The listing builds one solid part. Answer for the finished solid, in the listing's coordinates (mm). Face numbers are marked on the shaded views. A direction names the side the tool comes from. Round coordinates to 2 decimals unless told otherwise and drop trailing zeros. Loops run counter-clockwise (first coordinate to the right, second up) from the corner with the lowest first, then second, coordinate; pieces in that order, holes last. Notation, with made-up numbers: (72.25, 54) -> (93.25, 54) arc R16 ccw to (93.25, 85) -> close; hole circle Ø2 at (-37.5, 41). An arc over 180 degrees is marked (long way). One line per question, with ' | ' between items.
from build123d import *
from build123d.topology import SkipClean

# Parameters (mm, degrees)
SKETCH2_W                      = 63.5
SKETCH2_H                      = 63.5
BOSS_EXTRUDE1_DEPTH            = 80
CUT_EXTRUDE1_REACH             = 93.739
SKETCH4_R                      = 14.2875
CUT_EXTRUDE2_DEPTH             = 3.81
CUT_EXTRUDE3_DEPTH             = 62.22
CUT_EXTRUDE4_REACH             = 93.739
CUT_EXTRUDE4_DIRECTION_2_REACH = 93.739
FILLET2_R                      = 2.54
SKETCH9_W                      = 5
SKETCH9_H                      = 80
BOSS_EXTRUDE2_DEPTH            = 35
SKETCH10_R                     = 2.75
CUT_EXTRUDE6_DEPTH             = 119.642846392
CUT_EXTRUDE7_REACH             = 110.92
SKETCH11_R                     = 3
SKETCH12_W                     = 40
SKETCH12_H                     = 80
BOSS_EXTRUDE3_DEPTH            = 15
SKETCH13_R                     = 3
CUT_EXTRUDE8_DEPTH             = 10
FILLET3_R                      = 3.175
FILLET4_DEPTH                  = 80


with BuildPart() as part:
    # Sketch2 → Boss-Extrude1 (new body)
    with BuildSketch(Plane(origin=(0, 0, 0), x_dir=(1, 0, 0), z_dir=(0, 1, 0))):
        Rectangle(SKETCH2_W, SKETCH2_H)
    extrude(amount=BOSS_EXTRUDE1_DEPTH)

    # Sketch3 → Cut-Extrude1 (cut, up to next)
    with BuildSketch(Plane(origin=(0, 80, 0), x_dir=(1, 0, 0), z_dir=(0, 1, 0)), mode=Mode.PRIVATE) as cut_extrude1_sk1:
        with BuildLine():
            Line((9.525, 0), (14.2875, 0))
            ThreePointArc((14.2875, 0), (0, -14.2875), (-14.2875, 0))
            Line((-14.2875, 0), (-9.525, 0))
            ThreePointArc((-9.525, 0), (0, 9.525), (9.525, 0))
        make_face()
    cut_extrude1_tool1 = extrude(cut_extrude1_sk1.sketch, amount=-CUT_EXTRUDE1_REACH, mode=Mode.PRIVATE) & part.part
    add(cut_extrude1_tool1.solids().sort_by_distance((0, 80, 2.954161))[0], mode=Mode.SUBTRACT)

    # Sketch4 → Cut-Extrude2 (cut)
    with BuildSketch(Plane(origin=(0, 80, 0), x_dir=(1, 0, 0), z_dir=(0, 1, 0))):
        with Locations(Location((0, 0, 0), (0, 0, 270))):
            Circle(SKETCH4_R)
    extrude(amount=-CUT_EXTRUDE2_DEPTH, mode=Mode.SUBTRACT)

    # Sketch6 → Cut-Extrude3 (cut)
    with BuildSketch(Plane(origin=(0, 71.11, 0), x_dir=(1, 0, 0), z_dir=(0, 1, 0))):
        with BuildLine():
            Line((9.525, 0), (19.05, 31.75))
            Line((19.05, 31.75), (-19.05, 31.75))
            Line((-19.05, 31.75), (-9.525, 0))
            ThreePointArc((-9.525, 0), (0, 9.525), (9.525, 0))
        make_face()
    extrude(amount=-CUT_EXTRUDE3_DEPTH, mode=Mode.SUBTRACT)

    # Cut-Extrude4: up to this plane
    with SkipClean():  # the faces are left unmerged after this step: merging them gives an invalid solid
        cut_extrude4_end = Plane(origin=(-9.525, -49.595085442, 0), z_dir=(-0.9578262852211514, 0, 0.2873478855663456))
        # Sketch7 → Cut-Extrude4 (cut, up to the surface)
        with BuildSketch(Plane(origin=(0, 0, 0), x_dir=(0, 0, -1), z_dir=(1, 0, 0)), mode=Mode.PRIVATE) as cut_extrude4_sk1:
            Polygon((0, 8.89), (31.75, 8.89), (0, 0), align=None)
        cut_extrude4_tool1 = split(extrude(cut_extrude4_sk1.sketch, amount=-CUT_EXTRUDE4_REACH, mode=Mode.PRIVATE), bisect_by=cut_extrude4_end, keep=Keep.BOTH, mode=Mode.PRIVATE)
        add(cut_extrude4_tool1.solids().sort_by_distance((0, 5.926667, -10.583333))[0], mode=Mode.SUBTRACT)

    # Cut-Extrude4 direction 2: up to this plane
    cut_extrude4_direction_2_end = Plane(origin=(9.525, -49.595085442, 0), z_dir=(0.9578262852211514, 0, 0.2873478855663456))
    # Sketch7 → Cut-Extrude4 direction 2 (cut, up to the surface)
    with BuildSketch(Plane(origin=(0, 0, 0), x_dir=(0, 0, -1), z_dir=(1, 0, 0)), mode=Mode.PRIVATE) as cut_extrude4_direction_2_sk1:
        Polygon((0, 8.89), (31.75, 8.89), (0, 0), align=None)
    cut_extrude4_direction_2_tool1 = split(extrude(cut_extrude4_direction_2_sk1.sketch, amount=CUT_EXTRUDE4_DIRECTION_2_REACH, mode=Mode.PRIVATE), bisect_by=cut_extrude4_direction_2_end, keep=Keep.BOTH, mode=Mode.PRIVATE)
    add(cut_extrude4_direction_2_tool1.solids().sort_by_distance((0, 5.926667, -10.583333))[0], mode=Mode.SUBTRACT)

    # Fillet2
    # the kernel refuses this fillet: 2.54 mm, written as the material it adds along each edge
    with BuildSketch(Plane(origin=(7.700340927, 71.11, 6.082196911), x_dir=(-0.9578262852211513, 0, -0.2873478855663455), z_dir=(0.28734788556634555, 0, -0.9578262852211513))) as fillet2_piece_1_section:
        with BuildLine():
            CenterArc((FILLET2_R, -FILLET2_R), FILLET2_R, 90, 90)
            Line((0, -FILLET2_R), (0, 0))
            Line((0, 0), (FILLET2_R, 0))
        make_face()
    fillet2_piece_1 = extrude(amount=45.847973166, mode=Mode.PRIVATE)
    fillet2_piece_1 = split(fillet2_piece_1, bisect_by=Plane(origin=(7.700340927, 71.11, -31.75), z_dir=(0, 0, 1)), keep=Keep.TOP, mode=Mode.PRIVATE)
    fillet2_piece_1 = fillet2_piece_1 - Plane(origin=(0, 71.11, 0), x_dir=(-1, 0, 0), z_dir=(0, 1, 0)) * Cylinder(9.525, 102, mode=Mode.PRIVATE)
    fillet2_piece_1 = split(fillet2_piece_1, bisect_by=Plane(origin=(7.700340927, 71.11, 0), z_dir=(0, 0, -1)), keep=Keep.TOP, mode=Mode.PRIVATE)
    add(fillet2_piece_1)
    with BuildSketch(Plane(origin=(-20.874659073, 71.11, -37.832196911), x_dir=(0, -1, 0), z_dir=(0.28734788556634555, 0, 0.9578262852211513))) as fillet2_piece_2_section:
        with BuildLine():
            CenterArc((FILLET2_R, FILLET2_R), FILLET2_R, 180, 90)
            Line((0, FILLET2_R), (0, 0))
            Line((0, 0), (FILLET2_R, 0))
        make_face()
    fillet2_piece_2 = extrude(amount=45.847973166, mode=Mode.PRIVATE)
    fillet2_piece_2 = split(fillet2_piece_2, bisect_by=Plane(origin=(-20.874659073, 71.11, -31.75), z_dir=(0, 0, 1)), keep=Keep.TOP, mode=Mode.PRIVATE)
    fillet2_piece_2 = split(fillet2_piece_2, bisect_by=Plane(origin=(-20.874659073, 71.11, 0), z_dir=(0, 0, -1)), keep=Keep.TOP, mode=Mode.PRIVATE)
    fillet2_piece_2 = fillet2_piece_2 - Plane(origin=(0, 71.11, 0), x_dir=(-1, 0, 0), z_dir=(0, 1, 0)) * Cylinder(9.525, 102, mode=Mode.PRIVATE)
    add(fillet2_piece_2)
    with BuildSketch(Plane(origin=(-20.954648619, 10.667672044, -38.098828729), x_dir=(0.9607141016314922, 0.07483307171461691, -0.2672609704093551), z_dir=(0.2775399339309484, -0.2590372716688848, 0.9251331131031606))) as fillet2_piece_3_section:
        with BuildLine():
            CenterArc((FILLET2_R * 1.08072615035, FILLET2_R), FILLET2_R, 175.556407911, 94.443592089)
            Line((FILLET2_R * 0.0837320564804, FILLET2_R * 1.07747758898), (0, 0))
            Line((0, 0), (FILLET2_R * 1.08072615035, 0))
        make_face()
    fillet2_piece_3 = extrude(amount=52.848435405, mode=Mode.PRIVATE)
    fillet2_piece_3 = split(fillet2_piece_3, bisect_by=Plane(origin=(-20.954648619, 10.667672044, -31.75), z_dir=(0, 0, 1)), keep=Keep.TOP, mode=Mode.PRIVATE)
    fillet2_piece_3 = fillet2_piece_3 - Plane(origin=(0, 10.667672044, 0), x_dir=(-1, 0, 0), z_dir=(0, 1, 0)) * Cylinder(9.525, 117, mode=Mode.PRIVATE)
    fillet2_piece_3 = split(fillet2_piece_3, bisect_by=Plane(origin=(-20.954648619, 10.667672044, 0), z_dir=(0, 0, -1)), keep=Keep.TOP, mode=Mode.PRIVATE)
    add(fillet2_piece_3)
    with BuildSketch(Plane(origin=(20.954648619, 10.667672044, -38.098828729), x_dir=(-0.9607141016314922, 0.07483307171461691, -0.2672609704093551), z_dir=(-0.2775399339309484, -0.2590372716688848, 0.9251331131031606))) as fillet2_piece_4_section:
        with BuildLine():
            CenterArc((FILLET2_R * 1.08072615035, -FILLET2_R), FILLET2_R, 90, 94.443592089)
            Line((FILLET2_R * 0.0837320564804, -FILLET2_R * 1.07747758898), (0, 0))
            Line((0, 0), (FILLET2_R * 1.08072615035, 0))
        make_face()
    fillet2_piece_4 = extrude(amount=52.848435405, mode=Mode.PRIVATE)
    fillet2_piece_4 = split(fillet2_piece_4, bisect_by=Plane(origin=(20.954648619, 10.667672044, -31.75), z_dir=(0, 0, 1)), keep=Keep.TOP, mode=Mode.PRIVATE)
    fillet2_piece_4 = fillet2_piece_4 - Plane(origin=(0, 10.667672044, 0), x_dir=(-1, 0, 0), z_dir=(0, 1, 0)) * Cylinder(9.525, 117, mode=Mode.PRIVATE)
    fillet2_piece_4 = split(fillet2_piece_4, bisect_by=Plane(origin=(20.954648619, 10.667672044, 0), z_dir=(0, 0, -1)), keep=Keep.TOP, mode=Mode.PRIVATE)
    add(fillet2_piece_4)

    # Sketch9 → Boss-Extrude2 (add)
    with BuildSketch(Plane.XY.offset(31.75)):
        with Locations((-22.5, 40)):
            Rectangle(SKETCH9_W, SKETCH9_H)
        with Locations((22.5, 40)):
            Rectangle(SKETCH9_W, SKETCH9_H)
    extrude(amount=BOSS_EXTRUDE2_DEPTH)

    # Sketch10 → Cut-Extrude6 (cut, through all)
    with BuildSketch(Plane.ZY.offset(25)):
        with Locations(Location((56.75, 70, 0), (0, 0, 270))):
            Circle(SKETCH10_R)
        with Locations(Location((56.75, 10, 0), (0, 0, 270))):
            Circle(SKETCH10_R)
        with Locations(Location((56.75, 40, 0), (0, 0, 270))):
            Circle(SKETCH10_R)
    extrude(amount=-CUT_EXTRUDE6_DEPTH, mode=Mode.SUBTRACT)

    # Sketch11 → Cut-Extrude7 (cut, up to next)
    with BuildSketch(Plane.XZ, mode=Mode.PRIVATE) as cut_extrude7_sk1:
        with Locations(Location((26.042742751, -26.042742751, 0), (0, 0, 270))):
            Circle(SKETCH11_R)
    cut_extrude7_tool1 = extrude(cut_extrude7_sk1.sketch, amount=-CUT_EXTRUDE7_REACH, mode=Mode.PRIVATE) & part.part
    # Sketch11 → Cut-Extrude7 (cut, up to next)
    with BuildSketch(Plane.XZ, mode=Mode.PRIVATE) as cut_extrude7_sk2:
        with Locations(Location((26.042742751, 26.042742751, 0), (0, 0, 270))):
            Circle(SKETCH11_R)
    cut_extrude7_tool2 = extrude(cut_extrude7_sk2.sketch, amount=-CUT_EXTRUDE7_REACH, mode=Mode.PRIVATE) & part.part
    # Sketch11 → Cut-Extrude7 (cut, up to next)
    with BuildSketch(Plane.XZ, mode=Mode.PRIVATE) as cut_extrude7_sk3:
        with Locations(Location((-26.042742751, -26.042742751, 0), (0, 0, 270))):
            Circle(SKETCH11_R)
    cut_extrude7_tool3 = extrude(cut_extrude7_sk3.sketch, amount=-CUT_EXTRUDE7_REACH, mode=Mode.PRIVATE) & part.part
    # Sketch11 → Cut-Extrude7 (cut, up to next)
    with BuildSketch(Plane.XZ, mode=Mode.PRIVATE) as cut_extrude7_sk4:
        with Locations(Location((-26.042742751, 26.042742751, 0), (0, 0, 270))):
            Circle(SKETCH11_R)
    cut_extrude7_tool4 = extrude(cut_extrude7_sk4.sketch, amount=-CUT_EXTRUDE7_REACH, mode=Mode.PRIVATE) & part.part
    add(cut_extrude7_tool1.solids().sort_by_distance((26.042743, 0, -26.042743))[0], mode=Mode.SUBTRACT)
    add(cut_extrude7_tool2.solids().sort_by_distance((26.042743, 0, 26.042743))[0], mode=Mode.SUBTRACT)
    add(cut_extrude7_tool3.solids().sort_by_distance((-26.042743, 0, -26.042743))[0], mode=Mode.SUBTRACT)
    add(cut_extrude7_tool4.solids().sort_by_distance((-26.042743, 0, 26.042743))[0], mode=Mode.SUBTRACT)

    # Sketch12 → Boss-Extrude3 (add)
    with BuildSketch(Plane.XY.offset(31.75)):
        with Locations((0, 40)):
            Rectangle(SKETCH12_W, SKETCH12_H)
    extrude(amount=BOSS_EXTRUDE3_DEPTH)

    # Sketch13 → Cut-Extrude8 (cut)
    with BuildSketch(Plane(origin=(0, 0, -31.75), x_dir=(-1, 0, 0), z_dir=(0, 0, -1))):
        with Locations((-18.75, 75)):
            Circle(SKETCH13_R)
        with Locations(Location((18.75, 75, 0), (0, 0, 180))):
            Circle(SKETCH13_R)
        with Locations((18.75, 5)):
            Circle(SKETCH13_R)
        with Locations(Location((-18.75, 5, 0), (0, 0, 180))):
            Circle(SKETCH13_R)
    extrude(amount=-CUT_EXTRUDE8_DEPTH, mode=Mode.SUBTRACT)

    # Fillet3
    fillet3_edges = [part.edges().sort_by_distance(p)[0] for p in [
        (31.75, 40, 31.75),
        (-31.75, 40, 31.75),
        (-31.75, 40, -31.75),
        (31.75, 40, -31.75),
    ]]
    fillet(fillet3_edges, radius=FILLET3_R)

    # Fillet4: read off the stored shape, not the designer's step
    # Fillet4 outline → Fillet4 (add)
    with BuildSketch(Plane(origin=(0, 0, 0), x_dir=(1, 0, 0), z_dir=(0, 1, 0))):
        with BuildLine():
            Line((25, -31.75), (25, -36.624844719))
            ThreePointArc((25, -36.624844719), (26.168694859, -33.412197692), (29.128440367, -31.701392291))
            ThreePointArc((29.128440367, -31.701392291), (28.852785416, -31.737824728), (28.575, -31.75))
            Line((28.575, -31.75), (25, -31.75))
        make_face()
        with BuildLine():
            ThreePointArc((-28.575, -31.75), (-28.852785416, -31.737824728), (-29.128440367, -31.701392291))
            ThreePointArc((-29.128440367, -31.701392291), (-26.168694859, -33.412197692), (-25, -36.624844719))
            Line((-25, -36.624844719), (-25, -31.75))
            Line((-25, -31.75), (-28.575, -31.75))
        make_face()
    extrude(amount=FILLET4_DEPTH)


solid = part.part
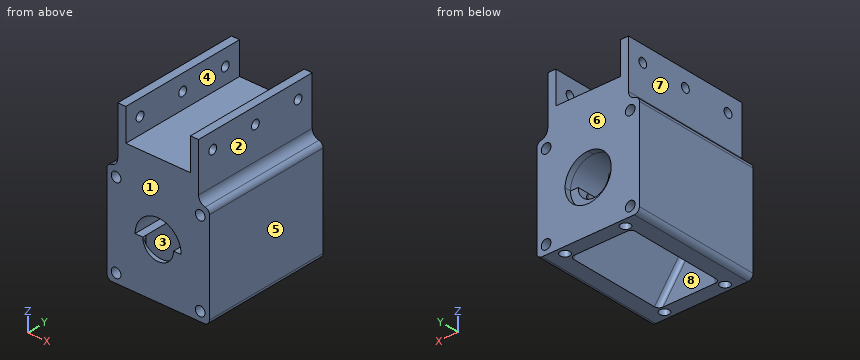
Q1. Find the intervals of material crossed by line 1 (Z direction, x = -21, y = 40); line 2 (X direction, y = 49, z = 60.5); line 3 (Y direction, x = 18.75, z = -25), in increasing order. Write a range as from..to.
Numbers:
line 1: -31.75..54, 59.5..66.75 | line 2: -25..-20, 20..25 | line 3: 0..2, 8..72, 78..80
Q2. A cutting plane is placed at D-D on z = 24.5. Give the vertices of the cut face in (x, y), plus the area to 3 significant figures.
Numbers:
outline: (-31.75, 0) -> (-28.62, 0) -> (-28.62, 80) -> (-31.75, 80) -> close; (-23.47, 0) -> (23.47, 0) -> (23.47, 80) -> (-23.47, 80) -> close; (28.62, 0) -> (31.75, 0) -> (31.75, 80) -> (28.62, 80) -> close | area: 4,260 mm^2
Q3. A cutting plane is placed at A-A on y = 39.5. Give the number of separate pieces and of enclosed holes in the cut face, plus the area to 3 significant figures.
Numbers:
separate pieces: 3 | enclosed holes: 4 | area: 3,590 mm^2
Q4. For a pull along Y with two mould halves and no side action, classify the marked faces 1, 2 and 3 as pulls with the +Y half, pulls with the -Y half, needs draft (parallel to the pull), parting line crosses it, or undercut.
Numbers:
face 1: pulls with the -Y half | face 2: needs draft | face 3: undercut
Q5. For the marked faces 4, 5, 6, 7 and 8, determine the directions among +Z, -Z, +X, -X, +Y, -Y from which every point of the face is accessible in a straight line to the end or side of a thin tool.
Numbers:
face 4: +Z, +Y, -Y | face 5: +Z, -Z, +X, +Y, -Y | face 6: +Z, -Z, +X, -X, +Y | face 7: +Z, -X, +Y, -Y | face 8: none
Q6. Given pin 1 Ø3 at (x, y) = (-18.5, 5.5) entering from -Z; pin 2 Ø6 at (y, z) = (60.5, 48.5) entering from +X; pin 3 Ø9.5 at (x, y) = (-18.75, 75) entering from -Z; pin 4 Ø4 at (x, y) = (3.5, 39) entering from +Z, each flat-ended and moving along its own axis, determine where each tip first touches the part or whether it passes through.
Numbers:
pin 1: z = -21.75 | pin 2: x = 25 | pin 3: z = -31.75 | pin 4: z = 46.75
Q7. A cutting plane is placed at C-C on x = 2. Give the vertices of the cut face in (y, z).
Numbers:
outline: (0, -31.75) -> (8.89, -31.75) -> (2.61, -9.31) -> (0, -9.31) -> close; (0, 14.15) -> (80, 14.15) -> (80, 46.75) -> (0, 46.75) -> close; (71.11, -31.75) -> (80, -31.75) -> (80, -14.15) -> (76.19, -14.15) -> (76.19, -9.31) -> (71.11, -9.31) -> close
